from build123d import *

# Parameters (mm, degrees)
SKETCH1_W           = 90
SKETCH1_H           = 20
BOSS_EXTRUDE1_DEPTH = 2
SKETCH2_R           = 4
SKETCH2_R_2         = 3.883174387
CUT_EXTRUDE1_DEPTH  = 2


with BuildPart() as part:
    # Sketch1 → Boss-Extrude1 (new body)
    with BuildSketch(Plane(origin=(0, 0, 0), x_dir=(1, 0, 0), z_dir=(0, 1, 0))):
        with Locations((45, 10)):
            Rectangle(SKETCH1_W, SKETCH1_H)
    extrude(amount=BOSS_EXTRUDE1_DEPTH)

    # Sketch2 → Cut-Extrude1 (cut)
    with BuildSketch(Plane(origin=(0, 2, 0), x_dir=(1, 0, 0), z_dir=(0, 1, 0))):
        with Locations(Location((10, 6, 0), (0, 0, 270))):
            Circle(SKETCH2_R)
        with Locations(Location((51, 14, 0), (0, 0, 270))):
            Circle(SKETCH2_R_2)
        with Locations(Location((80, 6, 0), (0, 0, 270))):
            Circle(SKETCH2_R)
        Polygon((0, 20), (0, 10), (45, 20), align=None)
        Polygon((90, 20), (60, 20), (90, 10), align=None)
    extrude(amount=-CUT_EXTRUDE1_DEPTH, mode=Mode.SUBTRACT)


solid = part.part
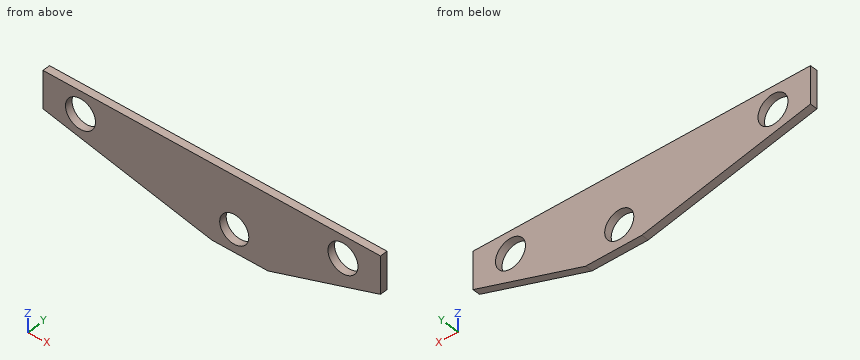
The model under review builds one solid part; all positions refer to its coordinate system, in mm. Give positions to 0.01 mm unless a question says otherwise; leave off trailing zeros. Write each loop counter-clockwise with the first axis right and the second up, starting at its lowest first coordinate (ties: lowest second). Pieces come first, ordered by that corner, then holes.
1. Add section A-A, the plane z = -6. Write out the cut boundary in (x, y), plus the area to 3 significant figures.
2. For P1, Ø7, axis at x = 80, z = -6, coming from the -Y side, flat-tipped, find the tip position at first contact; note if it passes through.
3. Add section C-C, the plane z = -14. Write out the cut boundary in (x, y), plus the area to 3 significant figures.
4. Wall thickness on L1, parallel to X at y = 0.8, z = -6; L2, parallel to X at y = 0.6, z = -8.5; L3, parallel to Z at x = 77.5, y = 1.7: over which ranges is each line inside the solid? List them lowest first.
5. Add section B-B, the plane x = 51. Write out the cut boundary in (y, z).
6. Add section D-D, the plane y = 1.6. Write out the cut boundary in (x, z), plus the area to 3 significant figures.
Worked answers:
1. outline: (0, 0) - (6, 0) - (6, 2) - (0, 2) - close; (14, 0) - (76, 0) - (76, 2) - (14, 2) - close; (84, 0) - (90, 0) - (90, 2) - (84, 2) - close
1. area: 148 mm2
2. P1: passes through
3. outline: (18, 0) - (47.12, 0) - (47.12, 2) - (18, 2) - close; (54.88, 0) - (78, 0) - (78, 2) - (54.88, 2) - close
3. area: 104 mm2
4. L1: x = 0 to 6, 14 to 76, 84 to 90
4. L2: x = 0 to 6.88, 13.12 to 76.88, 83.12 to 90
4. L3: z = -14.17 to -9.12, -2.88 to 0
5. outline: (0, -20) - (2, -20) - (2, -17.88) - (0, -17.88) - close; (0, -10.12) - (2, -10.12) - (2, 0) - (0, 0) - close
6. outline: (0, -10) - (45, -20) - (60, -20) - (90, -10) - (90, 0) - (0, 0) - close; hole circle Ø8 at (10, -6); hole circle Ø7.77 at (51, -14); hole circle Ø8 at (80, -6)
6. area: 1,280 mm2
